The figure shows three views and two pictorial views of one solid part (mm, origin at its lowest corner). Answer the questions. Give positions to 0.01 mm unless a question says otherwise; leave off trailing zeros. Loops run counter-clockwise (first coordinate to the right, second up) from the corner with the lowest first, then second, coordinate; pieces in that order, holes last. Notation, with made-up numbers: (32.25, 73.5) - (56.25, 73.5) arc R7 cw to (56.25, 81.5) - close; hole circle Ø8 at (62, -26.75). An arc over 180 degrees is marked (long way). Use CSV: the item, a comma, the result in double quotes.
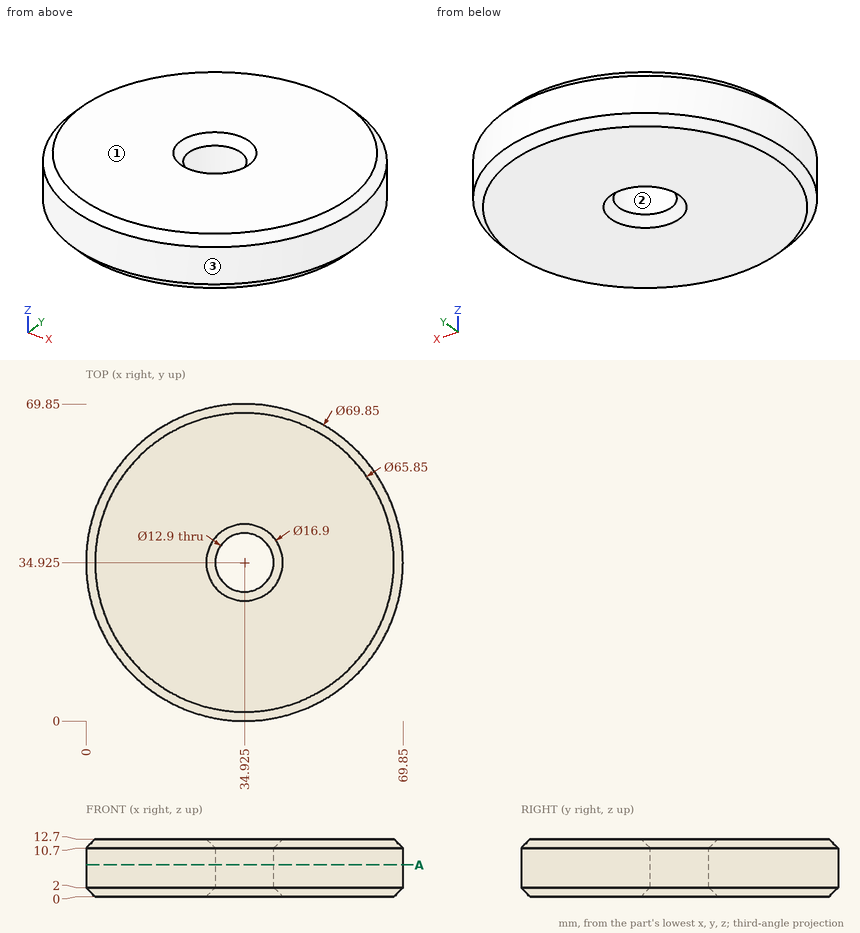
Item 1: The mould has two halves that part along Y. Classify the marked faces 1, 2 and 3: pulls with the +Y half, pulls with the -Y half, needs draft (parallel to the pull), parting line crosses it, or undercut.
Determined:
face 1,"needs draft"
face 2,"undercut"
face 3,"parting line crosses it"
Item 2: A cutting plane is placed at A-A on z = 7. Determine the outline of the cut face in (x, y) (3 decimals).
Determined:
outline,"circle Ø69.85 at (34.925, 34.925); hole circle Ø12.9 at (34.925, 34.925)"
Item 3: Find the intervals of material crossed by line 1 (Y direction, x = 35, z = 7.25); line 2 (Y direction, x = 31, z = 4.25); line 3 (X direction, y = 61.5, z = 10.25), in increasing order.
Determined:
line 1,"y = 0 to 28.48, 41.37 to 69.85"
line 2,"y = 0.22 to 29.81, 40.04 to 69.63"
line 3,"x = 12.26 to 57.59"
Item 4: Given P1, Ø15, axis at x = 34.925, y = 34.925, coming from the +Z side; P2, Ø2, axis at y = 52.5, z = 4, coming from the -X side; P3, Ø3, axis at x = 52.5, z = 2.5, coming from the +Y side, each flat-ended and moving along its own axis, determine where each tip first touches the part or whether it passes through.
Determined:
P1,"stops at z = 11.75"
P2,"stops at x = 4.18"
P3,"stops at y = 65.93"
